```python
from build123d import *
from OCP.BRepFilletAPI import BRepFilletAPI_MakeChamfer

# Parameters (mm, degrees)
SKETCH1_R           = 35
BOSS_EXTRUDE1_DEPTH = 72.403703
SKETCH2_R           = 28.211303246
CUT_EXTRUDE1_DEPTH  = 88.705736461
CHAMFER1_SIZE       = 3.533288
CHAMFER1_SIZE2      = 2.039945


with BuildPart() as part:
    # Sketch1 → Boss-Extrude1 (new body)
    with BuildSketch(Plane(origin=(0, 0, 0), x_dir=(1, 0, 0), z_dir=(0, 1, 0))):
        with Locations(Location((0, 0, 0), (0, 0, 270))):
            Circle(SKETCH1_R)
    extrude(amount=BOSS_EXTRUDE1_DEPTH)

    # Sketch2 → Cut-Extrude1 (cut, through all)
    with BuildSketch(Plane(origin=(0, 0, 0), x_dir=(1, 0, 0), z_dir=(0, 1, 0))):
        with Locations(Location((0, 0, 0), (0, 0, 270))):
            Circle(SKETCH2_R)
    extrude(amount=CUT_EXTRUDE1_DEPTH, mode=Mode.SUBTRACT)

    # Chamfer1: one chamfer whose edges measure the first distance from different faces: ONE call of the kernel's chamfer builder (chamfer() names one face for all edges)
    chamfer1_edges_1 = [part.edges().sort_by_distance(p)[0] for p in [
        (0, 0, -35),
    ]]
    chamfer1_side_1 = [part.faces().sort_by_distance(p)[0] for p in [
        (0, 0, -34.010050506),
    ]]
    chamfer1_edges_2 = [part.edges().sort_by_distance(p)[0] for p in [
        (0, 72.403703, -35),
    ]]
    chamfer1_side_2 = [part.faces().sort_by_distance(p)[0] for p in [
        (0, 36.2018515, -35),
    ]]
    chamfer1_edges_3 = [part.edges().sort_by_distance(p)[0] for p in [
        (0, 0, -28.211303246),
    ]]
    chamfer1_side_3 = [part.faces().sort_by_distance(p)[0] for p in [
        (0, 36.2018515, -28.211303246),
    ]]
    chamfer1_edges_4 = [part.edges().sort_by_distance(p)[0] for p in [
        (0, 72.403703, -28.211303246),
    ]]
    chamfer1_side_4 = [part.faces().sort_by_distance(p)[0] for p in [
        (0, 72.403703, -34.010050506),
    ]]
    chamfer1 = BRepFilletAPI_MakeChamfer(part.part.solid().wrapped)
    for e in chamfer1_edges_1:
        chamfer1.Add(CHAMFER1_SIZE, CHAMFER1_SIZE2, e.wrapped, chamfer1_side_1[0].wrapped)  # the first distance lies on this face
    for e in chamfer1_edges_2:
        chamfer1.Add(CHAMFER1_SIZE, CHAMFER1_SIZE2, e.wrapped, chamfer1_side_2[0].wrapped)  # the first distance lies on this face
    for e in chamfer1_edges_3:
        chamfer1.Add(CHAMFER1_SIZE, CHAMFER1_SIZE2, e.wrapped, chamfer1_side_3[0].wrapped)  # the first distance lies on this face
    for e in chamfer1_edges_4:
        chamfer1.Add(CHAMFER1_SIZE, CHAMFER1_SIZE2, e.wrapped, chamfer1_side_4[0].wrapped)  # the first distance lies on this face
    add(Compound.cast(chamfer1.Shape()), mode=Mode.REPLACE)


solid = part.part
```
Geometry check sheet. Reference: the model listing, model coordinates, mm. Give positions to 0.01 mm unless a question says otherwise; leave off trailing zeros. Loops run counter-clockwise (first coordinate to the right, second up) from the corner with the lowest first, then second, coordinate; pieces in that order, holes last. Notation, with made-up numbers: M 8.5,72 L 22.5,72 A13 cw 22.5,79 Z; hole C 49.5,64 d9. An arc over 180 degrees is marked long. Write item = value, one per line. Start each with the question number.
1. Go/stop test with flat-tipped pins: P1, Ø12, axis at y = 21, z = -26, coming from the -X side; P2, Ø10, axis at y = 63.5, z = 0, coming from the -X side; P3, Ø2, axis at x = -11.5, z = 23, coming from the +Y side; P4, Ø1.5, axis at x = -0.5, y = 44, coming from the +Z side. Record where each tip stops, or that it passes through.
2. Section check A-A, the plane x = 0. Enter the section's corners in (y, z).
3. Thickness scan on probe 1 along X at (y, z) = (48.5, 0); probe 2 along Z at (x, y) = (17, 47). Record the ranges inside material, lowest first.
4. Section check B-B, the plane z = 0. Enter the section's corners in (x, y).
5. Draft check along Z on faces 1 (the face through (-27.54, 36.48, -6.12)), 2 (the face through (26, 0, -16)), 3 (the face through (-20.116, 72.232, -26.235)). Enter one of: +Z half, -Z half, draft (parallel to the pull), parting line (faces both ways), or undercut.
6. Section check C-C, the plane y = 29. Enter the section's corners in (x, z), plus the area to 3 significant figures.
Values follow:
q1.P1 = -28.72
q1.P2 = -35
q1.P3 = through
q1.P4 = 35
q2.outline = M 0,-31.47 L 2.04,-35 L 68.87,-35 L 72.4,-32.96 L 72.4,-31.74 L 70.36,-28.21 L 3.53,-28.21 L 0,-30.25 Z; M 0,30.25 L 3.53,28.21 L 70.36,28.21 L 72.4,31.74 L 72.4,32.96 L 68.87,35 L 2.04,35 L 0,31.47 Z
q3.probe_1 = -35 to -28.21, 28.21 to 35
q3.probe_2 = -30.59 to -22.51, 22.51 to 30.59
q4.outline = M -35,2.04 L -31.47,0 L -30.25,0 L -28.21,3.53 L -28.21,70.36 L -31.74,72.4 L -32.96,72.4 L -35,68.87 Z; M 28.21,3.53 L 30.25,0 L 31.47,0 L 35,2.04 L 35,68.87 L 32.96,72.4 L 31.74,72.4 L 28.21,70.36 Z
q5.face_1 = undercut
q5.face_2 = draft
q5.face_3 = parting line
q6.outline = C 0,0 d70; hole C 0,0 d56.42
q6.area = 1,350 mm^2
